Input: dimensioned drawing with shaded views. Units: mm. Origin: part minimum x, y, z. A direction names the side the tool comes from. Coordinates: 2 decimals unless noted, no trailing zeros. Order: outer loops, then holes, each group sorted by start corner. A loop starts at its lowest first (then second) coordinate and runs counter-clockwise, first axis right, second up.
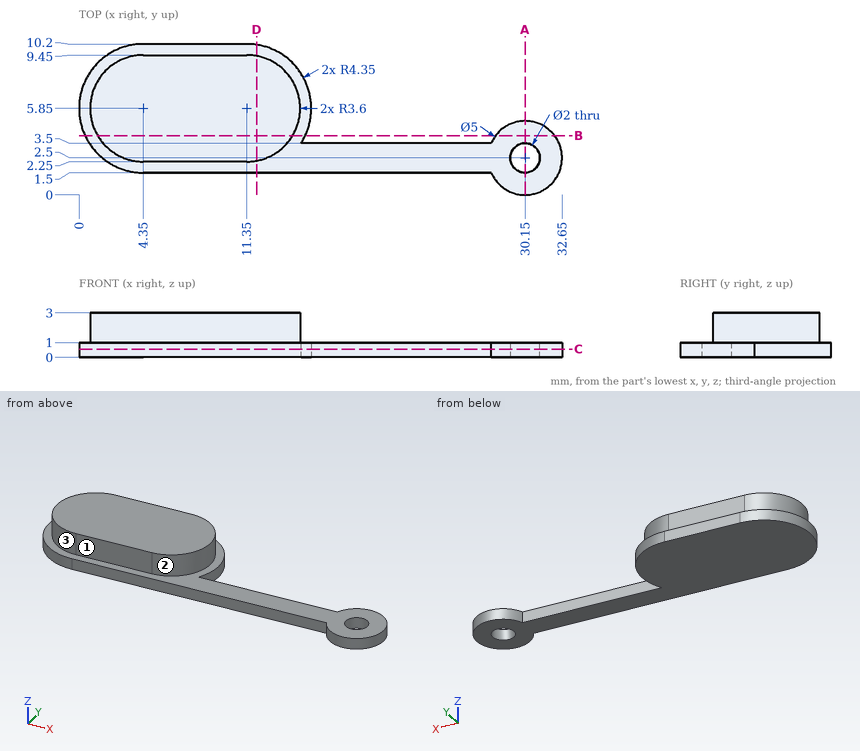
1. Section query D-D, the plane x = 12. Output: boundary loops of the cut face in (y, z), plus the area to 3 significant figures.
2. Contact query for flat-ended pins moving along their axis: P1, Ø1.6, axis at x = 7, z = 2.5, coming from the -Y side; P2, Ø1.1, axis at x = 10.5, z = 0.5, coming from the -Y side. Output: stop coordinate, or through.
3. Section query C-C, the plane z = 0.55. Output: boundary loops of the cut face in (x, y).
4. Section query B-B, the plane y = 4. Output: boundary loops of the cut face in (x, z).
5. Material intervals for line 1 along Y through (x, z) = (30.15, 0.55); line 2 along Z through (x, y) = (30.5, 0.75); line 3 along Y through (x, z) = (25.5, 0.2), sorted ascending.
6. Section query A-A, the plane x = 30.15. Output: boundary loops of the cut face in (y, z).
7. Access query for the marked faces 1, 2 and 3. Directions: +Z, -Z, +X, -X, +Y, -Y. A direction counts if a zero-diameter tool reaches every point of the face in a straight line with its end or side. Return the directions, or none.
Answer key:
1. outline: (1.5, 0) - (10.15, 0) - (10.15, 1) - (9.39, 1) - (9.39, 3) - (2.31, 3) - (2.31, 1) - (1.5, 1) - close
1. area: 22.8 mm2
2. P1: stops at y = 2.25
2. P2: stops at y = 1.5
3. outline: (4.35, 1.5) - (27.86, 1.5) arc R2.5 ccw (long way) to (27.86, 3.5) - (15.01, 3.5) arc R4.35 ccw to (11.35, 10.2) - (4.35, 10.2) arc R4.35 ccw to start; hole circle Ø2 at (30.15, 2.5)
4. outline: (0.41, 0) - (15.29, 0) - (15.29, 1) - (14.44, 1) - (14.44, 3) - (1.26, 3) - (1.26, 1) - (0.41, 1) - close; (28.15, 0) - (32.15, 0) - (32.15, 1) - (28.15, 1) - close
5. line 1: y = 0 to 1.5, 3.5 to 5
5. line 2: z = 0 to 1
5. line 3: y = 1.5 to 3.5
6. outline: (0, 0) - (1.5, 0) - (1.5, 1) - (0, 1) - close; (3.5, 0) - (5, 0) - (5, 1) - (3.5, 1) - close
7. face 1: +Z, +X, -X, -Y
7. face 2: +Z, +X
7. face 3: +Z, -X
